For this review, use the dimensioned drawing (mm, ordinates from the lowest corner) and the shaded views. Round coordinates to 2 decimals unless told otherwise and drop trailing zeros. Loops run counter-clockwise (first coordinate to the right, second up) from the corner with the lowest first, then second, coordinate; pieces in that order, holes last. Notation, with made-up numbers: M -8.75,61 L -0.75,61 A15 ccw -0.75,76 Z; hole C 48.5,51.5 d1. An arc over 180 degrees is marked long. Answer as a JSON object with one key per item and string values. Group by question number.
Item 1: Consider section D-D (x = 6). Give the boundary of the cut face in (y, z), and give its area (3 significant figures).
Item 2: Consider section C-C (z = 1.5). Give the boundary of the cut face in (x, y), and give its area (4 significant figures).
Item 3: To check wall thickness, follow line 1 (X direction, y = 1, z = 1.5); line 2 (Z direction, x = 39.5, y = 0.9); line 3 (X direction, y = 1.6, z = 49). State the ranges of each line that lie inside material, in increasing order.
Item 4: Insertion check: P1, Ø1.8, axis at x = 39.5, z = 49, coming from the -Y side. The pin has a flat end and moves straight along its axis. Give the tip position at first contact, or say it passes through.
Item 5: Consider section B-B (x = 39.5). Give the boundary of the cut face in (y, z), and give its area (3 significant figures).
Item 6: Consider section A-A (z = 21). Give the boundary of the cut face in (x, y), and give its area (4 significant figures).
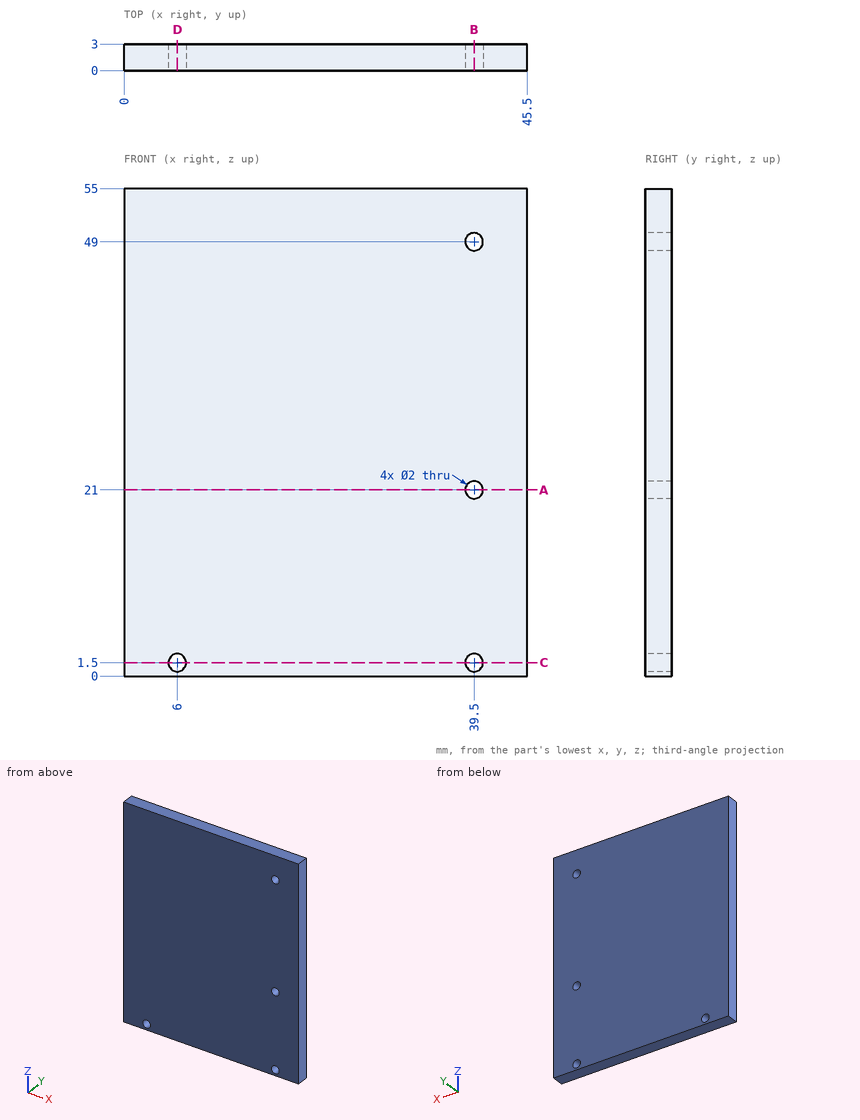
Geometry results:
{
 "1": {"outline": "M 0,0 L 3,0 L 3,0.5 L 0,0.5 Z; M 0,2.5 L 3,2.5 L 3,55 L 0,55 Z", "area": "159 mm^2"},
 "2": {"outline": "M 0,0 L 5,0 L 5,3 L 0,3 Z; M 7,0 L 38.5,0 L 38.5,3 L 7,3 Z; M 40.5,0 L 45.5,0 L 45.5,3 L 40.5,3 Z", "area": "124.5 mm^2"},
 "3": {"line 1": "x = 0 to 5, 7 to 38.5, 40.5 to 45.5", "line 2": "z = 0 to 0.5, 2.5 to 20, 22 to 48, 50 to 55", "line 3": "x = 0 to 38.5, 40.5 to 45.5"},
 "4": {"P1": "passes through"},
 "5": {"outline": "M 0,0 L 3,0 L 3,0.5 L 0,0.5 Z; M 0,2.5 L 3,2.5 L 3,20 L 0,20 Z; M 0,22 L 3,22 L 3,48 L 0,48 Z; M 0,50 L 3,50 L 3,55 L 0,55 Z", "area": "147 mm^2"},
 "6": {"outline": "M 0,0 L 38.5,0 L 38.5,3 L 0,3 Z; M 40.5,0 L 45.5,0 L 45.5,3 L 40.5,3 Z", "area": "130.5 mm^2"}
}
